Work out the finished part from the listing and answer in its coordinate system (mm). Give positions to 0.01 mm unless a question says otherwise; leave off trailing zeros. Loops run counter-clockwise (first coordinate to the right, second up) from the corner with the lowest first, then second, coordinate; pieces in that order, holes last. Notation, with made-up numbers: (75, -37) - (108, -37) arc R36 ccw to (108, 2) - close; hole circle Ø9 at (41, 43.25). An arc over 180 degrees is marked (long way). One line per item, written item: value.
from build123d import *

# Parameters (mm, degrees)
F1_W     = 240
F1_H     = 240
F1_W_2   = 6
F1_H_2   = 6
F1_W_3   = 208
F1_H_3   = 208
F2_DEPTH = 3
F3_DEPTH = 25
F8_W     = 216
F8_H     = 16
F8_W_2   = 208
F8_H_2   = 208
F9_DEPTH = 3.001


with BuildPart() as f2:
    # F1 (on Front) → F2 (new body)
    with BuildSketch(Plane.XZ):
        with Locations((120, 120)):
            Rectangle(F1_W, F1_H)
        with Locations((6, 234)):
            Rectangle(F1_W_2, F1_H_2, mode=Mode.SUBTRACT)
        with Locations((120, 120)):
            Rectangle(F1_W_3, F1_H_3, mode=Mode.SUBTRACT)
        with Locations((6, 234)):
            Rectangle(F1_W_2, F1_H_2)
    extrude(amount=F2_DEPTH)

    # F1 (on Front) → F3 (cut)
    with BuildSketch(Plane.XZ):
        with Locations((6, 234)):
            Rectangle(F1_W_2, F1_H_2)
    extrude(amount=F3_DEPTH, mode=Mode.SUBTRACT)

    # F5: F2 across plane


with BuildPart() as f2_1:
    add(f2.part)
    add(f2.part.mirror(Plane(origin=(120, -1.5, 120), x_dir=(0, -1, 0), z_dir=(-1, 0, 0))), mode=Mode.INTERSECT)

    # F7: F2 across plane


with BuildPart() as f2_2:
    add(f2_1.part)
    add(f2_1.part.mirror(Plane(origin=(120, -1.5, 120), x_dir=(1, 0, 0), z_dir=(0, 0, 1))), mode=Mode.INTERSECT)

    # F8 (on face) → F9 (cut, through all)
    with BuildSketch(Plane.XZ.offset(3)):
        with Locations((120, 248)):
            Rectangle(F8_W, F8_H)
        with Locations((120, 120)):
            Rectangle(F8_W_2, F8_H_2)
        Polygon((228, 240), (12, 240), (12, 16), (16, 16), (16, 224), (224, 224), (224, 16), (228, 16), align=None)
    extrude(amount=-F9_DEPTH, mode=Mode.SUBTRACT)


solid = f2_2.part
1. A flat-ended cylindrical pin translates along its axis: pin 1 Ø0.9 at (y, z) = (-1.5, 130.5) entering from -X. Find the tip coordinate at first contact, or state that the pin passes through.
Output:
pin 1: stops at x = 0
2. Section B-B (z = 182.5) is taken. Write down the section's boundary in (x, y).
Output:
outline: (0, -3) - (12, -3) - (12, 0) - (0, 0) - close; (228, -3) - (240, -3) - (240, 0) - (228, 0) - close
3. Find the intervals of material crossed by line 1 along X through (y, z) = (-2.6, 208.5); line 2 along Z through (x, y) = (74, -2.3), in increasing order.
Output:
line 1: x = 0 to 12, 228 to 240
line 2: z = 0 to 16
4. Section C-C (x = 61) is taken. Write down the section's boundary in (y, z), and give its area (3 significant figures).
Output:
outline: (-3, 0) - (0, 0) - (0, 16) - (-3, 16) - close
area: 48.0 mm²
5. Section A-A (y = -0.8) is taken. Write down the section's boundary in (x, z), and give its area (3 significant figures).
Output:
outline: (0, 0) - (240, 0) - (240, 240) - (228, 240) - (228, 16) - (12, 16) - (12, 240) - (0, 240) - close; hole (3, 3) - (9, 3) - (9, 9) - (3, 9) - close; hole (3, 231) - (9, 231) - (9, 237) - (3, 237) - close; hole (231, 3) - (237, 3) - (237, 9) - (231, 9) - close; hole (231, 231) - (237, 231) - (237, 237) - (231, 237) - close
area: 9,070 mm²
